```python
from build123d import *

# Parameters (mm, degrees)
ESBO_O1_R                = 50
ESBO_O1_R_2              = 40
RESSALTO_EXTRUS_O1_DEPTH = 10
ESBO_O2_R                = 3
CORTE_EXTRUS_O1_DEPTH    = 10
RESSALTO_EXTRUS_O2_START = -10
RESSALTO_EXTRUS_O2_DEPTH = 10
FILETE3_SIZE             = 5


with BuildPart() as part:
    # Esboço1 → Ressalto-extrusão1 (new body)
    with BuildSketch(Plane.XY):
        Circle(ESBO_O1_R)
        Circle(ESBO_O1_R_2, mode=Mode.SUBTRACT)
    extrude(amount=RESSALTO_EXTRUS_O1_DEPTH)

    # Esboço2 → Corte-extrusão1 (cut)
    with BuildSketch(Plane.XY.offset(10)):
        with Locations((45, 0)):
            Circle(ESBO_O2_R)
        with Locations((42.797543233, -13.905764747)):
            Circle(ESBO_O2_R)
        with Locations((36.405764747, -26.450336353)):
            Circle(ESBO_O2_R)
        with Locations((26.450336353, -36.405764747)):
            Circle(ESBO_O2_R)
        with Locations((13.905764747, -42.797543233)):
            Circle(ESBO_O2_R)
        with Locations((0, -45)):
            Circle(ESBO_O2_R)
        with Locations((-13.905764747, -42.797543233)):
            Circle(ESBO_O2_R)
        with Locations((-26.450336353, -36.405764747)):
            Circle(ESBO_O2_R)
        with Locations((-36.405764747, -26.450336353)):
            Circle(ESBO_O2_R)
        with Locations((-42.797543233, -13.905764747)):
            Circle(ESBO_O2_R)
        with Locations((-45, 0)):
            Circle(ESBO_O2_R)
        with Locations((-42.797543233, 13.905764747)):
            Circle(ESBO_O2_R)
        with Locations((-36.405764747, 26.450336353)):
            Circle(ESBO_O2_R)
        with Locations((-26.450336353, 36.405764747)):
            Circle(ESBO_O2_R)
        with Locations((-13.905764747, 42.797543233)):
            Circle(ESBO_O2_R)
        with Locations((0, 45)):
            Circle(ESBO_O2_R)
        with Locations((13.905764747, 42.797543233)):
            Circle(ESBO_O2_R)
        with Locations((26.450336353, 36.405764747)):
            Circle(ESBO_O2_R)
        with Locations((36.405764747, 26.450336353)):
            Circle(ESBO_O2_R)
        with Locations((42.797543233, 13.905764747)):
            Circle(ESBO_O2_R)
    extrude(amount=-CORTE_EXTRUS_O1_DEPTH, mode=Mode.SUBTRACT)

    # Esboço3 → Ressalto-extrusão2 (add)
    with BuildSketch(Plane.XY.offset(10).offset(RESSALTO_EXTRUS_O2_START)):
        with BuildLine():
            Line((-39.686269666, -5), (-5, -5))
            Line((-5, -5), (-5, -39.686269666))
            ThreePointArc((-5, -39.686269666), (0, -40), (5, -39.686269666))
            Line((5, -39.686269666), (5, -5))
            Line((5, -5), (39.686269666, -5))
            ThreePointArc((39.686269666, -5), (40, 0), (39.686269666, 5))
            Line((39.686269666, 5), (5, 5))
            Line((5, 5), (5, 39.686269666))
            ThreePointArc((5, 39.686269666), (0, 40), (-5, 39.686269666))
            Line((-5, 39.686269666), (-5, 5))
            Line((-5, 5), (-39.686269666, 5))
            ThreePointArc((-39.686269666, 5), (-40, 0), (-39.686269666, -5))
        make_face()
    extrude(amount=RESSALTO_EXTRUS_O2_DEPTH)

    # Filete3
    # a fillet whose section is not a circle: 5 mm, written as the material it adds along each edge
    with BuildSketch(Plane(origin=(-39.686269666, -5, 0), x_dir=(0.20605308678190473, -0.9785408143903089, 0), z_dir=(0, 0, 1)), Plane(origin=(39.686269666, 5, 0), x_dir=(-0.206053086781907, 0.9785408143903084, 0), z_dir=(0, 0, 1)), Plane(origin=(5, -39.686269666, 0), x_dir=(0.9785408143903085, 0.2060530867819072, 0), z_dir=(0, 0, 1)), Plane(origin=(-5, 39.686269666, 0), x_dir=(-0.9785408143903084, -0.206053086781907, 0), z_dir=(0, 0, 1))) as filete3_piece_1:
        with BuildLine():
            Bezier((6.569548591, 0), (-0.115998395, -0.550873396), (1.266247732, 6.013377943), weights=[1, 1, 1])
            Line((1.266247732, 6.013377943), (0, 0))
            ThreePointArc((0, 0), (3.284774296, -0.135099927), (6.569548591, 0))
        make_face()
    extrude(amount=10)
    with BuildSketch(Plane(origin=(5, 5, 0), x_dir=(1, 0, 0), z_dir=(0, 0, 1)), Plane(origin=(5, -5, 0), x_dir=(0, -1, 0), z_dir=(0, 0, 1)), Plane(origin=(-5, -5, 0), x_dir=(-1, 0, 0), z_dir=(0, 0, 1)), Plane(origin=(-5, 5, 0), x_dir=(0, 1, 0), z_dir=(0, 0, 1))) as filete3_piece_2:
        with BuildLine():
            Bezier((FILETE3_SIZE, 0), (0, 0), (0, FILETE3_SIZE), weights=[1, 1, 1])
            Line((0, FILETE3_SIZE), (0, 0))
            Line((0, 0), (FILETE3_SIZE, 0))
        make_face()
    extrude(amount=10)
    with BuildSketch(Plane(origin=(5, 39.686269666, 0), x_dir=(0.9785408143903086, -0.20605308678190615, 0), z_dir=(0, 0, 1)), Plane(origin=(-5, -39.686269666, 0), x_dir=(-0.9785408143903087, 0.20605308678190526, 0), z_dir=(0, 0, 1)), Plane(origin=(39.686269666, -5, 0), x_dir=(-0.20605308678190642, -0.9785408143903086, 0), z_dir=(0, 0, 1)), Plane(origin=(-39.686269666, 5, 0), x_dir=(0.206053086781904, 0.9785408143903089, 0), z_dir=(0, 0, 1))) as filete3_piece_3:
        with BuildLine():
            Bezier((6.569548591, 0), (-0.115998395, 0.550873396), (1.266247732, -6.013377943), weights=[1, 1, 1])
            Line((1.266247732, -6.013377943), (0, 0))
            ThreePointArc((0, 0), (3.284774296, 0.135099927), (6.569548591, 0))
        make_face()
    extrude(amount=10)


solid = part.part
```
Read the model definition and answer for the solid it produces. Units are mm, in the model's axes. Coordinates: 2 decimals unless noted, no trailing zeros. Write each loop counter-clockwise with the first axis right and the second up, starting at its lowest first coordinate (ties: lowest second). Pieces come first, ordered by that corner, then holes. Notation, with made-up numbers: (51, -4.75) -> (79, -4.75) arc R30 cw to (79, 18.25) -> close; hole circle Ø7 at (-36, -1). An arc over 180 degrees is marked (long way). Answer as a JSON object with one key per item and string values.
Q1. The part is cut by section B-B on y = -7. Give the number of separate pieces and of enclosed holes in the cut face, then the cut area to 3 significant figures.
The answers:
{"separate pieces": "3", "enclosed holes": "0", "area": "337 mm2"}
Q2. Consider line 1 (X direction, y = -23, z = 5.25); line 2 (X direction, y = 25, z = 7.5); line 3 (X direction, y = -22, z = 4.25). Determine where each line is inside the solid, lowest interval first. Write a range as [from, to].
The answers:
{"line 1": "x = [-44.4, -32.73], [-5, 5], [32.73, 44.4]", "line 2": "x = [-43.3, -39.03], [-33.78, -31.22], [-5, 5], [31.22, 33.78], [39.03, 43.3]", "line 3": "x = [-44.9, -33.41], [-5, 5], [33.41, 44.9]"}
Q3. The part is cut by section A-A on x = 0. Give the vertices of the cut face in (y, z), then the cut area to 3 significant figures.
The answers:
{"outline": "(-50, 0) -> (-48, 0) -> (-48, 10) -> (-50, 10) -> close; (-42, 0) -> (42, 0) -> (42, 10) -> (-42, 10) -> close; (48, 0) -> (50, 0) -> (50, 10) -> (48, 10) -> close", "area": "880 mm2"}
Q4. Determine the mould class of faces 1 (the cylindrical face through (47.69, 15.02, 4.93)), 2 (the cylindrical face through (0, 48, 5)), 3 (the flat face through (0, -3, 10)) for opening direction X: pulls with the +X half, pulls with the -X half, needs draft (parallel to the pull), parting line crosses it, or undercut.
The answers:
{"face 1": "parting line crosses it", "face 2": "undercut", "face 3": "needs draft"}
Q5. Flat-ended cylindrical pins translate along their axes: pin 1 Ø1.5 at (y, z) = (26, 8.5) entering from -X; pin 2 Ø4 at (x, y) = (-36, -1.5) entering from -Z; pin 3 Ø1.5 at (y, z) = (5.5, 7.5) entering from +X; pin 4 Ø4 at (x, z) = (38, 3.5) entering from +Y. Find the tip coordinate at first contact, or state that the pin passes through.
The answers:
{"pin 1": "stops at x = -43.16", "pin 2": "stops at z = 0", "pin 3": "stops at x = 49.77", "pin 4": "stops at y = 34.7"}
